Build history of the part. All positions in model axes, mm. Face numbers are marked on the shaded views. A direction names the side the tool comes from. Give positions to 0.01 mm unless a question says otherwise; leave off trailing zeros. Order: outer loops, then holes, each group sorted by start corner. A loop starts at its lowest first (then second) coordinate and runs counter-clockwise, first axis right, second up. Notation, with made-up numbers: M -7.5,39.5 L 39.5,39.5 A27 cw 39.5,69.5 Z; hole C 63.25,31 d3. An arc over 180 degrees is marked long. Use CSV: the item, a comma, the result in double quotes. Start each with the question number.
Item 1: Which spindle directions (+Z, -Z, +X, -X, +Y, -Y) get a long thin tool onto all of the face, cutting with end or side? Do the marked faces 4, 5 and 6. Say none if no direction does.
Item 2: Two-plate mould, pull along Z, no slides. Class the marked faces 1, 2 and 3: pulls with the +Z half, pulls with the -Z half, needs draft (parallel to the pull), parting line crosses it, or undercut.
Item 3: Band-saw the part on A-A on y = 0. Write the cut outline in (x, z), plus the area to 3 significant figures.
Item 4: Wall check: line 1 along Y through (x, z) = (59, 0); line 2 along Y through (x, z) = (36, 27); line 3 along X through (y, z) = (-25.5, 0.5). Give the ranges that are in metal, low to high.
Item 5: Band-saw the part on B-B on z = 0. Write the cut outline in (x, y).
Item 6: Pin check, flat tips, straight feed: P1, Ø12, axis at x = 61, y = 4.5, coming from the -Z side; P2, Ø2, axis at x = 55.5, z = -14.5, coming from the -Y side; P3, Ø10, axis at x = 59, y = -22.5, coming from the +Z side. Stop position of each tip, or through.
Item 7: Band-saw the part on C-C on z = -27.5. Write the cut outline in (x, y), plus the area to 3 significant figures.
Item 8: Band-saw the part on D-D on x = 62. Write the cut outline in (y, z).
Autodesk Inventor part; units mm, degrees
ref_plane "YZ Plane" through (0, 0, 0) normal (1, 0, 0) x (0, 1, 0)
ref_plane "XZ Plane" through (0, 0, 0) normal (0, 1, 0) x (-1, 0, 0)
ref_plane "XY Plane" through (0, 0, 0) normal (0, 0, 1) x (1, 0, 0)
sketch "Skizze1" plane through (0, 0, 0) normal (0, 0, 1) x (1, 0, 0)
  line L0 (0, 0) -> (0, 18)
  line L1 (0, 18) -> (17, 18)
  line L2 (17, 18) -> (17, 31.5)
  line L3 (17, 31.5) -> (70, 31.5)
  line L4 (70, 31.5) -> (70, 0)
  line L5 (70, 0) -> (0, 0)
  dimension "d0" = 70
  dimension "d1" = 36
  dimension "d2" = 17
  dimension "d3" = 63
revolve "Umdrehung1" add sketch "Skizze1" angle 360 about axis through (70, 0, 0) along (-1, 0, 0)
sketch "Skizze2" plane through (70, 0, 0) normal (1, 0, 0) x (0, 0, -1)
  circle A0 centre (0, 0) radius 22.5
  dimension "d5" = 45
extrude "Extrusion1" cut sketch "Skizze2" against normal blind 40
sketch "Skizze8" plane through (70, 0, 0) normal (1, 0, 0) x (0, 0, -1)
  line L0 (0, 0) -> (0, 31.8712) construction
  point P0 (-27.5, 0)
  point P1 (27.5, 0)
  dimension "d38" = 55
hole "Bohrung5" at (70, 0, 27.5) at (70, 0, -27.5) direction (-1, 0, 0) diameter 4.917 depth 53
fillet "Rundung1" radius 2 1 edges at (0, -18, 0)
sketch "Skizze3" plane through (30, 0, 0) normal (1, 0, 0) x (0, 0, -1)
  line L0 (0, 0) -> (0, 13.1561) construction
  point P0 (-10, 0)
  point P1 (10, 0)
  dimension "d8" = 20
sketch "Skizze4" plane through (30, 0, 0) normal (1, 0, 0) x (0, 0, -1)
  circle A0 centre (10, 0) radius 2
  point P0 (0, 0)
  point P1 (10, 0)
sketch "Skizze6" plane through (0, 0, 0) normal (-1, 0, 0) x (0, 0, 1)
  circle A0 centre (10, 0) radius 2
  point P0 (0, 0)
  point P1 (10, 0)
sketch "Skizze5" plane through (0, 0, 0) normal (-1, 0, 0) x (0, 0, 1)
  circle A0 centre (-10, 0) radius 2
  point P0 (0, 0)
  point P1 (-10, 0)
properties part number "Zylinder" material "Stahl, galvanisiert"
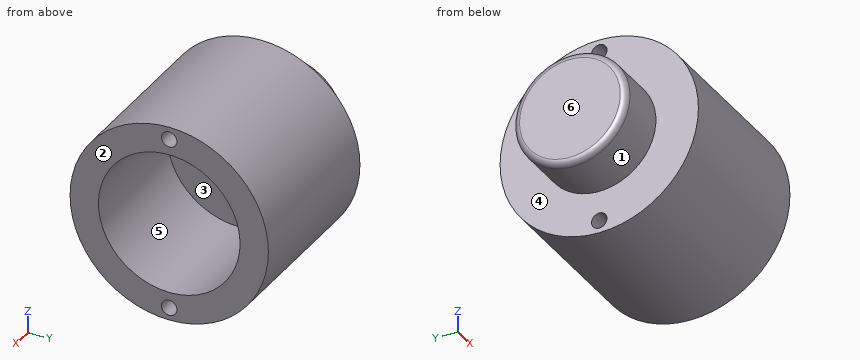
Model answer:
1,face 4,"-X"
1,face 5,"+X"
1,face 6,"+Z, -Z, -X, +Y, -Y"
2,face 1,"parting line crosses it"
2,face 2,"needs draft"
2,face 3,"undercut"
3,outline,"M 0,-16 A2 ccw 2,-18 L 17,-18 L 17,-25.04 L 70,-25.04 L 70,-22.5 L 30,-22.5 L 30,22.5 L 70,22.5 L 70,25.04 L 17,25.04 L 17,18 L 2,18 A2 ccw 0,16 Z; M 17,-31.5 L 70,-31.5 L 70,-29.96 L 17,-29.96 Z; M 17,29.96 L 70,29.96 L 70,31.5 L 17,31.5 Z"
3,area,"1,630 mm^2"
4,line 1,"y = -31.5 to -22.5, 22.5 to 31.5"
4,line 2,"y = -16.22 to -2.41, 2.41 to 16.22"
4,line 3,"x = 17 to 70"
5,outline,"M 0,-16 A2 ccw 2,-18 L 17,-18 L 17,-31.5 L 70,-31.5 L 70,-22.5 L 30,-22.5 L 30,22.5 L 70,22.5 L 70,31.5 L 17,31.5 L 17,18 L 2,18 A2 ccw 0,16 Z"
6,P1,"stops at z = -31.5"
6,P2,"stops at y = -28.46"
6,P3,"stops at z = 26.19"
7,outline,"M 17,-15.36 L 70,-15.36 L 70,-2.46 L 17,-2.46 Z; M 17,2.46 L 70,2.46 L 70,15.36 L 17,15.36 Z"
7,area,"1,370 mm^2"
8,outline,"C 0,0 d63; hole C 0,0 d45; hole C 0,-27.5 d4.92; hole C 0,27.5 d4.92"
